```python
from build123d import *

# Parameters (mm, degrees)
CUT_EXTRUDE2_DEPTH = 2
CHAMFER1_SIZE      = 0.5
CHAMFER2_SIZE      = 0.25


with BuildPart() as part:
    # Sketch1 → Revolve1 (revolve)
    with BuildSketch(Plane(origin=(0, 0, 0), x_dir=(0, 0, -1), z_dir=(1, 0, 0))):
        Polygon((0, 0), (0, 5), (3, 5), (3, 2.65), (11.98, 2.65), (11.98, 0), align=None)
    revolve(axis=Axis((0, 0, 0), (0, 0, -1)))

    # Sketch2 → Cut-Extrude2 (cut)
    with BuildSketch(Plane.XY):
        Polygon((0, 2.886751346), (-2.5, 1.443375673), (-2.5, -1.443375673), (0, -2.886751346), (2.5, -1.443375673), (2.5, 1.443375673), align=None)
    extrude(amount=-CUT_EXTRUDE2_DEPTH, mode=Mode.SUBTRACT)

    # Chamfer1
    chamfer1_edges = [part.edges().sort_by_distance(p)[0] for p in [
        (0, -5, 0),
    ]]
    chamfer(chamfer1_edges, length=CHAMFER1_SIZE)

    # Chamfer2
    chamfer2_edges = [part.edges().sort_by_distance(p)[0] for p in [
        (0, -2.65, -11.98),
    ]]
    chamfer(chamfer2_edges, length=CHAMFER2_SIZE)


solid = part.part
```
For this review, take the finished solid that the model builds, in its own axes (mm). A direction names the side the tool comes from. Give positions to 0.01 mm unless a question says otherwise; leave off trailing zeros. Write each loop counter-clockwise with the first axis right and the second up, starting at its lowest first coordinate (ties: lowest second). Pieces come first, ordered by that corner, then holes.
Item 1: Insertion check: P1, Ø2, axis at y = -4, z = -1.5, coming from the +X side; P2, Ø1.5, axis at x = 1, z = -7, coming from the -Y side; P3, Ø3, axis at y = 1, z = -8.5, coming from the -X side. Each pin has a flat end and moves straight along its axis. Give the tip position at first contact, or say it passes through.
Item 2: Take a section at C-C (z = -8). Give the boundary of the cut face in (x, y), and give its area (3 significant figures).
Item 3: Machinability: for faces 1 (the face through (0, 0, -11.98)), 2 (the face through (-2, 2, -3)), 3 (the face through (-1.233, 2.175, -0.986)), which of the approach directions +Z, -Z, +X, -X, +Y, -Y give a long, thin tool a straight path to every point of the face, cutting with its end or side? Answer none if there is none.
Item 4: The part is to be moulded in two halves that separate along Y. For faces 4 (the face through (1.233, -2.175, -0.986)), 5 (the face through (-2, -2, 0)), 6 (the face through (2.5, 0, -1)), 7 (the face through (-1.01, 2.45, -7.43)), say which applies: +Y half, -Y half, draft (parallel to the pull), parting line (faces both ways), or undercut.
Item 5: Take a section at A-A (z = -1.75). Give the boundary of the cut face in (x, y).
Item 6: Take a section at B-B (y = 0). Give the boundary of the cut face in (x, z).
Item 7: Wall thickness on probe 1 along Z at (x, y) = (4.25, 0.25); probe 2 along Z at (x, y) = (-2, -0.25); probe 3 along X at (y, z) = (-1, -5.25): over which ranges is each line inside the solid? List them lowest first.
Established:
1. P1: stops at x = 4
1. P2: stops at y = -2.64
1. P3: stops at x = -2.65
2. outline: circle Ø5.3 at (0, 0)
2. area: 22.1 mm2
3. face 1: -Z, +X, -X, +Y, -Y
3. face 2: -Z
3. face 3: +Z
4. face 4: undercut
4. face 5: draft
4. face 6: undercut
4. face 7: parting line
5. outline: circle Ø10 at (0, 0); hole (-2.5, -1.44) - (0, -2.89) - (2.5, -1.44) - (2.5, 1.44) - (0, 2.89) - (-2.5, 1.44) - close
6. outline: (-5, -3) - (-2.65, -3) - (-2.65, -11.73) - (-2.4, -11.98) - (2.4, -11.98) - (2.65, -11.73) - (2.65, -3) - (5, -3) - (5, -0.5) - (4.5, 0) - (2.5, 0) - (2.5, -2) - (-2.5, -2) - (-2.5, 0) - (-4.5, 0) - (-5, -0.5) - close
7. probe 1: z = -3 to 0
7. probe 2: z = -11.98 to -2
7. probe 3: x = -2.45 to 2.45
